Build history of the part. All positions in model axes, mm. Coordinates: 2 decimals unless noted, no trailing zeros. Order: outer loops, then holes, each group sorted by start corner. A loop starts at its lowest first (then second) coordinate and runs counter-clockwise, first axis right, second up. Notation, with made-up numbers: (-7, 12) - (26, 12) arc R33 ccw to (26, 47) - close; hole circle Ø4 at (-35, 40). An arc over 180 degrees is marked (long way). Answer as CSV lines item,"result". Start each with the question number.
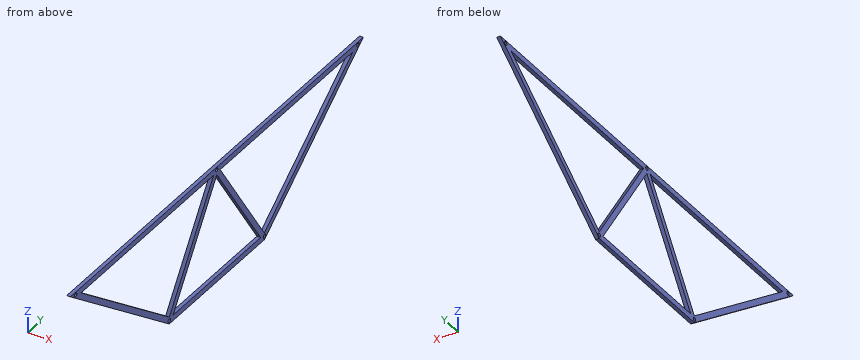
from build123d import *

# Parameters (mm, degrees)
BOSS_EXTRUDE2_DEPTH = 10
SKETCH6_R           = 5
CUT_EXTRUDE3_DEPTH  = 10


with BuildPart() as part:
    # Sketch4 → Boss-Extrude2 (new body)
    with BuildSketch(Plane.YZ):
        Polygon((-185.986121811, -292.5), (-190.986121811, -300), (190.986121811, -300), (185.986121811, -292.5), align=None)
        Polygon((600, 0), (9.013878189, 0), (14.013878189, -7.5), (577.5, -7.5), (201.842585459, -289.243060906), (197.5, -292.5), (195, -292.5), (200, -300), align=None)
        Polygon((-200, -300), (-600, 0), (-9.013878189, 0), (0, 0), (9.013878189, 0), (600, 0), (200, -300), (190.986121811, -300), (195.986121811, -307.5), (202.5, -307.5), (622.5, 7.5), (-622.5, 7.5), (-202.5, -307.5), (-195.986121811, -307.5), (-190.986121811, -300), align=None)
        Polygon((-9.013878189, 0), (-600, 0), (-200, -300), (-195, -292.5), (-197.5, -292.5), (-201.842585459, -289.243060906), (-577.5, -7.5), (-14.013878189, -7.5), align=None)
        Polygon((-5, -7.5), (-14.013878189, -7.5), (-201.842585459, -289.243060906), (-197.5, -292.5), (-195, -292.5), align=None)
        Polygon((-5, -7.5), (-195, -292.5), (-185.986121811, -292.5), (0, -13.520817283), (185.986121811, -292.5), (195, -292.5), (5, -7.5), align=None)
        Polygon((-195, -292.5), (-200, -300), (-190.986121811, -300), (-185.986121811, -292.5), align=None)
        Polygon((190.986121811, -300), (-190.986121811, -300), (-195.986121811, -307.5), (195.986121811, -307.5), align=None)
        Polygon((14.013878189, -7.5), (5, -7.5), (195, -292.5), (197.5, -292.5), (201.842585459, -289.243060906), align=None)
        Polygon((185.986121811, -292.5), (190.986121811, -300), (200, -300), (195, -292.5), align=None)
        Polygon((0, 0), (-9.013878189, 0), (-14.013878189, -7.5), (-5, -7.5), align=None)
        Polygon((9.013878189, 0), (0, 0), (5, -7.5), (14.013878189, -7.5), align=None)
        Polygon((5, -7.5), (0, 0), (-5, -7.5), align=None)
    extrude(amount=BOSS_EXTRUDE2_DEPTH)

    # Sketch6 → Cut-Extrude3 (cut)
    with BuildSketch(Plane.YZ.offset(10)):
        with Locations(Location((0, 0, 0), (0, 0, 270))):
            Circle(SKETCH6_R)
        with Locations(Location((-600, 0, 0), (0, 0, 270))):
            Circle(SKETCH6_R)
        with Locations(Location((-202.274610117, -298.294042412, 0), (0, 0, 270))):
            Circle(SKETCH6_R)
        with Locations(Location((202.274610117, -298.294042412, 0), (0, 0, 270))):
            Circle(SKETCH6_R)
        with Locations(Location((600, 0, 0), (0, 0, 270))):
            Circle(SKETCH6_R)
    extrude(amount=-CUT_EXTRUDE3_DEPTH, mode=Mode.SUBTRACT)


solid = part.part
(1) Probe L1, parallel to Y at x = 5.5, z = -279; L2, parallel to Y at x = 6.5, z = -285; L3, parallel to Y at x = 4.5, z = -9. List the from-to ranges inside material, lowest first. Write a range as [from, to].
(2) Band-saw the part on C-C on y = 532. List the corners of the cut face in (x, z) (3 decimals), plus the area to 4 significant figures.
(3) Drop flat-ended pins along their axis: pin 1 Ø3 at (x, y) = (3.5, -225) entering from -Z; pin 2 Ø11.5 at (y, z) = (-202.27, -298.29) entering from -X; pin 3 Ø8 at (y, z) = (202.27, -298.29) entering from +X; pin 4 Ø4 at (x, y) = (6.5, 444.5) entering from -Z. Give the stop position or say it passes through.
(4) Band-saw the part on A-A on y = -142. List the corners of the cut face in (x, z).
(5) Band-saw the part on B-B on z = -92. List the corners of the cut face in (x, y), plus the area to 3 significant figures.
(6) Band-saw the part on D-D on x = 2.5. State how many separate pieces and enclosed holes the cut face has, plus the area to 3 significant figures.
Filled in:
1,L1,"y = [-240.5, -215.5], [-195.01, -176.99], [176.99, 195.01], [215.5, 240.5]"
1,L2,"y = [-232.5, -207.5], [-199.01, -180.99], [180.99, 199.01], [207.5, 232.5]"
1,L3,"y = [-600.5, -575.5], [-15.01, 15.01], [575.5, 600.5]"
2,outline,"(0, -60.375) - (10, -60.375) - (10, -41.625) - (0, -41.625) - close; (0, -7.5) - (10, -7.5) - (10, 7.5) - (0, 7.5) - close"
2,area,"337.5 mm^2"
3,pin 1,"stops at z = -291.75"
3,pin 2,"stops at x = 0"
3,pin 3,"passes through"
3,pin 4,"stops at z = -127.5"
4,outline,"(0, -307.5) - (10, -307.5) - (10, -292.5) - (0, -292.5) - close; (0, -226.52) - (10, -226.52) - (10, -199.48) - (0, -199.48) - close; (0, -7.5) - (10, -7.5) - (10, 7.5) - (0, 7.5) - close"
5,outline,"(0, -489.83) - (10, -489.83) - (10, -464.83) - (0, -464.83) - close; (0, -70.35) - (10, -70.35) - (10, -52.32) - (0, -52.32) - close; (0, 52.32) - (10, 52.32) - (10, 70.35) - (0, 70.35) - close; (0, 464.83) - (10, 464.83) - (10, 489.83) - (0, 489.83) - close"
5,area,"861 mm^2"
6,separate pieces,"1"
6,enclosed holes,"8"
6,area,"48,800 mm^2"
